CAD build for the part. Positions are in the model's coordinates, mm. A direction names the side the tool comes from. Give positions to 0.01 mm unless a question says otherwise; leave off trailing zeros. Loops run counter-clockwise (first coordinate to the right, second up) from the corner with the lowest first, then second, coordinate; pieces in that order, holes last. Notation, with made-up numbers: M 78.5,20.25 L 132.5,20.25 A27 cw 132.5,59.25 Z; hole C -11.75,-2 d8. An arc over 180 degrees is marked long. One line per question, with ' | ' between items.
```python
from build123d import *

# Parameters (mm, degrees)
SKETCH1_W                                   = 107.1
SKETCH1_H                                   = 45.3
BOSS_EXTRUDE1_DEPTH                         = 3
SKETCH2_W                                   = 110.9
SKETCH2_H                                   = 49.1
SKETCH2_W_2                                 = 103.1
SKETCH2_H_2                                 = 41.3
BOSS_EXTRUDE2_DEPTH                         = 2
SKETCH5_W                                   = 44.185299266
SKETCH5_H                                   = 3
BOSS_EXTRUDE3_DEPTH                         = 1.9
SKETCH6_W                                   = 53.3
SKETCH6_H                                   = 5
BOSS_EXTRUDE4_DEPTH                         = 2
FILLET1_R                                   = 2
BOSS_EXTRUDE5_DEPTH                         = 3
FILLET2_R                                   = 3
CBORE_FOR_M3_CHEESE_HEAD_SCREW1_D           = 3.4
CBORE_FOR_M3_CHEESE_HEAD_SCREW1_CBORE_D     = 6.5
CBORE_FOR_M3_CHEESE_HEAD_SCREW1_CBORE_DEPTH = 2
SKETCH9_R                                   = 2.55
SKETCH9_W                                   = 4.3
SKETCH9_H                                   = 8.6
CUT_EXTRUDE1_DEPTH                          = 65.457156313
BOSS_EXTRUDE6_START                         = 5
SKETCH11_R                                  = 3.55
SKETCH11_R_2                                = 2.55
SKETCH11_W                                  = 2
SKETCH11_H                                  = 15
BOSS_EXTRUDE6_DEPTH                         = 5
CUT_EXTRUDE2_START                          = -1
SKETCH12_R                                  = 3.55
CUT_EXTRUDE2_DEPTH                          = 1


with BuildPart() as part:
    # Sketch1 → Boss-Extrude1 (new body)
    with BuildSketch(Plane(origin=(0, 0, 0), x_dir=(1, 0, 0), z_dir=(0, 1, 0))):
        Rectangle(SKETCH1_W, SKETCH1_H)
    extrude(amount=BOSS_EXTRUDE1_DEPTH)

    # Sketch2 → Boss-Extrude2 (add)
    with BuildSketch(Plane.XZ):
        Rectangle(SKETCH2_W, SKETCH2_H)
        Rectangle(SKETCH2_W_2, SKETCH2_H_2, mode=Mode.SUBTRACT)
    extrude(amount=BOSS_EXTRUDE2_DEPTH)

    # Sweep3: sweep along a path in Sketch4
    with BuildLine(Plane(origin=(0, 0, 0), x_dir=(1, 0, 0), z_dir=(0, 1, 0))) as sweep3_path:
        Line((55.45, 24.55), (-55.45, 24.55))
        Line((-55.45, 24.55), (-55.45, -24.55))
        Line((-55.45, -24.55), (55.45, -24.55))
    # Sketch3 → Sweep3 (sweep)
    with BuildSketch(Plane(origin=(55.45, 0, 0), x_dir=(0, 0, -1), z_dir=(1, 0, 0))):
        Polygon((-22.65, 3), (-25.65, 3), (-22.65, 0), (-22.092649633, 0), (-22.092649633, 3), align=None)
    sweep(path=sweep3_path.line, transition=Transition.RIGHT)

    # Sketch5 → Boss-Extrude3 (add)
    with BuildSketch(Plane(origin=(53.55, 0, 0), x_dir=(0, 0, -1), z_dir=(1, 0, 0))):
        with Locations((0, 1.5)):
            Rectangle(SKETCH5_W, SKETCH5_H)
    extrude(amount=BOSS_EXTRUDE3_DEPTH)

    # Sketch6 → Boss-Extrude4 (add)
    with BuildSketch(Plane(origin=(55.45, 0, 0), x_dir=(0, 0, -1), z_dir=(1, 0, 0))):
        with Locations((0, 0.5)):
            Rectangle(SKETCH6_W, SKETCH6_H)
    extrude(amount=BOSS_EXTRUDE4_DEPTH)

    # Fillet1
    fillet1_edges = [part.edges().sort_by_distance(p)[0] for p in [
        (57.45, 0.5, 26.65),
        (57.45, 0.5, -26.65),
    ]]
    fillet(fillet1_edges, radius=FILLET1_R - 0.0001)  # a hair under: the kernel refuses the full size

    # Sketch7 → Boss-Extrude5 (add)
    with BuildSketch(Plane(origin=(57.45, 0, 0), x_dir=(0, 0, -1), z_dir=(1, 0, 0))):
        with BuildLine():
            Line((-10, -2), (10, -2))
            ThreePointArc((10, -2), (0, -12), (-10, -2))
        make_face()
    extrude(amount=-BOSS_EXTRUDE5_DEPTH)

    # Fillet2
    fillet2_edges = [part.edges().sort_by_distance(p)[0] for p in [
        (55.95, -2, -10),
        (55.95, -2, 10),
    ]]
    fillet(fillet2_edges, radius=FILLET2_R)

    # CBORE for M3 Cheese Head Screw1 (through all)
    with Locations(Plane(origin=(57.45, -7, 0), x_dir=(0, 0, 1), z_dir=(1, 0, 0))):
        with Locations((0, 0)):
            CounterBoreHole(CBORE_FOR_M3_CHEESE_HEAD_SCREW1_D / 2, CBORE_FOR_M3_CHEESE_HEAD_SCREW1_CBORE_D / 2, CBORE_FOR_M3_CHEESE_HEAD_SCREW1_CBORE_DEPTH)

    # Sketch9 → Cut-Extrude1 (cut, through all)
    with BuildSketch(Plane.XZ):
        with Locations(Location((20, 0, 0), (0, 0, 270))):
            Circle(SKETCH9_R)
        with Locations(Location((-30, 0, 0), (0, 0, 270))):
            Circle(SKETCH9_R)
        with Locations((30, 0)):
            Rectangle(SKETCH9_W, SKETCH9_H)
        with Locations((-20, 0)):
            Rectangle(SKETCH9_W, SKETCH9_H)
    extrude(amount=-CUT_EXTRUDE1_DEPTH, mode=Mode.SUBTRACT)

    # Sketch11 → Boss-Extrude6 (add)
    # profile 1 of 6: a face of its own
    with BuildSketch(Plane.XZ.offset(BOSS_EXTRUDE6_START)):
        with Locations(Location((-30, 0, 0), (0, 0, 90))):
            Circle(SKETCH11_R)
        with Locations(Location((-30, 0, 0), (0, 0, 270))):
            Circle(SKETCH11_R_2, mode=Mode.SUBTRACT)
    # profile 2 of 6: a face of its own
    with BuildSketch(Plane.XZ.offset(BOSS_EXTRUDE6_START)):
        with Locations(Location((20, 0, 0), (0, 0, 90))):
            Circle(SKETCH11_R)
        with Locations(Location((20, 0, 0), (0, 0, 270))):
            Circle(SKETCH11_R_2, mode=Mode.SUBTRACT)
    # profile 3 of 6: a face of its own
    with BuildSketch(Plane.XZ.offset(BOSS_EXTRUDE6_START)):
        with Locations((-15.25, 0)):
            Rectangle(SKETCH11_W, SKETCH11_H)
    # profile 4 of 6: a face of its own
    with BuildSketch(Plane.XZ.offset(BOSS_EXTRUDE6_START)):
        with Locations((-24.75, 0)):
            Rectangle(SKETCH11_W, SKETCH11_H)
    # profile 5 of 6: a face of its own
    with BuildSketch(Plane.XZ.offset(BOSS_EXTRUDE6_START)):
        with Locations((34.516532033, 0)):
            Rectangle(SKETCH11_W, SKETCH11_H)
    # profile 6 of 6: a face of its own
    with BuildSketch(Plane.XZ.offset(BOSS_EXTRUDE6_START)):
        with Locations((25.483467967, 0)):
            Rectangle(SKETCH11_W, SKETCH11_H)
    extrude(amount=-BOSS_EXTRUDE6_DEPTH)

    # Sketch12 → Cut-Extrude2 (cut)
    with BuildSketch(Plane(origin=(0, 3, 0), x_dir=(1, 0, 0), z_dir=(0, 1, 0)).offset(CUT_EXTRUDE2_START)):
        with Locations(Location((-30, 0, 0), (0, 0, 270))):
            Circle(SKETCH12_R)
        with Locations(Location((20, 0, 0), (0, 0, 270))):
            Circle(SKETCH12_R)
    extrude(amount=CUT_EXTRUDE2_DEPTH, mode=Mode.SUBTRACT)


solid = part.part
```
Item 1: Drop flat-ended pins along their axis: P1, Ø5, axis at y = -10.5, z = 11, coming from the -X side; P2, Ø3.5, axis at x = -19, y = 1, coming from the -Z side; P3, Ø1, axis at x = 15.5, z = 17.5, coming from the -Y side; P4, Ø3, axis at y = 0, z = -24, coming from the -X side. Give the stop position or say it passes through.
Conclusion:
P1: through | P2: z = -25.4 | P3: y = 0 | P4: x = -55.45
Item 2: Saw through at B-B on z = 6. Give the cut face in (x, y), and give its area (3 significant figures).
Conclusion:
outline: M -56.55,3 L -53.55,0 L -55.45,0 L -55.45,-2 L -51.55,-2 L -51.55,0 L -25.75,0 L -25.75,-5 L -23.75,-5 L -23.75,0 L -16.25,0 L -16.25,-5 L -14.25,-5 L -14.25,0 L 24.48,0 L 24.48,-5 L 26.48,-5 L 26.48,0 L 33.52,0 L 33.52,-5 L 35.52,-5 L 35.52,0 L 51.55,0 L 51.55,-2 L 54.45,-2 L 54.45,-10 L 57.45,-10 L 57.45,3 Z | area: 421 mm²
Item 3: Saw through at A-A on x = 20. Give the cut face in (y, z).
Conclusion:
outline: M -5,-3.55 L 0,-3.55 L 0,-20.65 L -2,-20.65 L -2,-24.55 L 0,-24.55 L 0,-22.65 L 3,-25.65 L 3,-3.55 L 2,-3.55 L 2,-2.55 L -5,-2.55 Z; M -5,2.55 L 2,2.55 L 2,3.55 L 3,3.55 L 3,25.65 L 0,22.65 L 0,24.55 L -2,24.55 L -2,20.65 L 0,20.65 L 0,3.55 L -5,3.55 Z
Item 4: 3-axis set-ups, long thin cutter, end or side, ignore diameter. For faces 4 (the flat face through (-15, -3, -7.5)), 5 (the flat face through (55.45, -5.6, 1.4)), 6 (the flat face through (54.45, -5, 0)), 7 (the cylindrical face through (23.52, 2.49, -0.46)), 8 (the flat face through (27.85, 1, 0)): which of +Z, -Z, +X, -X, +Y, -Y reach the whole face in a straight line?
Conclusion:
face 4: -Y | face 5: +X | face 6: +Z, -Z, -Y | face 7: +Y | face 8: +Y, -Y
Item 5: Saw through at C-C on y = -7. Give the cut face in (x, z), and give its area (3 significant figures).
Conclusion:
outline: M 54.45,-8.66 L 57.45,-8.66 L 57.45,-3.25 L 55.45,-3.25 L 55.45,-1.7 L 54.45,-1.7 Z; M 54.45,1.7 L 55.45,1.7 L 55.45,3.25 L 57.45,3.25 L 57.45,8.66 L 54.45,8.66 Z | area: 35.6 mm²
Item 6: Mould opens along X. For faces 1 (the cylindrical face through (56, -12, 0)), 2 (the cylindrical face through (-27.47, -1.55, 0.33)), 3 (the cylindrical face through (56.88, 0.54, -26.05)) say: pulls with the +X half, pulls with the -X half, needs draft (parallel to the pull), parting line crosses it, or undercut.
Conclusion:
face 1: needs draft | face 2: undercut | face 3: pulls with the +X half
Item 7: Drill centre lines: line 1 along X through (y, z) = (-1.25, -16); line 2 along X through (y, z) = (2.25, 0); line 3 along Z through (x, y) = (-41, -0.25). Where is each one in solid material? Low to high. Write a range as [from, to].
Conclusion:
line 1: [-55.45, -51.55], [51.55, 57.45] | line 2: [-55.8, -33.55], [-26.45, -22.15], [-17.85, 16.45], [23.55, 27.85], [32.15, 57.45] | line 3: [-24.55, -20.65], [20.65, 24.55]
Item 8: Saw through at D-D on x = 41. Give the cut face in (y, z).
Conclusion:
outline: M -2,-24.55 L 0,-24.55 L 0,-22.65 L 3,-25.65 L 3,25.65 L 0,22.65 L 0,24.55 L -2,24.55 L -2,20.65 L 0,20.65 L 0,-20.65 L -2,-20.65 Z
